from build123d import *

# Parameters (mm, degrees)
SKETCH1_W           = 304.8
SKETCH1_H           = 50.8
SKETCH1_R           = 2.6
SKETCH1_R_2         = 4.05
BOSS_EXTRUDE1_DEPTH = 3.175


with BuildPart() as part:
    # Sketch1 → Boss-Extrude1 (new body)
    with BuildSketch(Plane(origin=(0, 0, 0), x_dir=(1, 0, 0), z_dir=(0, 1, 0))):
        with Locations((152.4, 25.4)):
            Rectangle(SKETCH1_W, SKETCH1_H)
        with Locations(Location((19.185127899, 44.45, 0), (0, 0, 270))):
            Circle(SKETCH1_R, mode=Mode.SUBTRACT)
        with Locations(Location((19.185127899, 20, 0), (0, 0, 270))):
            Circle(SKETCH1_R_2, mode=Mode.SUBTRACT)
        with Locations(Location((99.185127899, 20, 0), (0, 0, 270))):
            Circle(SKETCH1_R_2, mode=Mode.SUBTRACT)
        with Locations(Location((99.185127899, 44.45, 0), (0, 0, 270))):
            Circle(SKETCH1_R, mode=Mode.SUBTRACT)
        with Locations(Location((179.185127899, 20, 0), (0, 0, 270))):
            Circle(SKETCH1_R_2, mode=Mode.SUBTRACT)
        with Locations(Location((179.185127899, 44.45, 0), (0, 0, 270))):
            Circle(SKETCH1_R, mode=Mode.SUBTRACT)
        with Locations(Location((259.185127899, 20, 0), (0, 0, 270))):
            Circle(SKETCH1_R_2, mode=Mode.SUBTRACT)
        with Locations(Location((259.185127899, 44.45, 0), (0, 0, 270))):
            Circle(SKETCH1_R, mode=Mode.SUBTRACT)
    extrude(amount=BOSS_EXTRUDE1_DEPTH)


solid = part.part
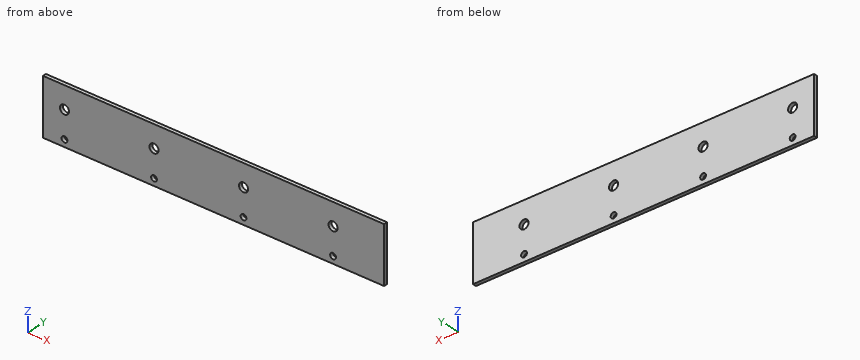
Read the model definition and answer for the solid it produces. Units are mm, in the model's axes. Coordinates: 2 decimals unless noted, no trailing zeros. Loops run counter-clockwise (first coordinate to the right, second up) from the corner with the lowest first, then second, coordinate; pieces in that order, holes last. Notation, with made-up numbers: (-8.5, 61) -> (-0.5, 61) arc R21 ccw to (-0.5, 82) -> close; hole circle Ø2 at (37.25, 9). An arc over 180 degrees is marked (long way). Answer in a Markdown table with one row per item.
Item 1: A cutting plane is placed at A-A on z = -44.45. Determine the outline of the cut face in (x, y) (3 decimals), plus the area to 3 significant figures.
Returned:
| item | result |
|---|---|
| outline | (0, 0) -> (16.585, 0) -> (16.585, 3.175) -> (0, 3.175) -> close; (21.785, 0) -> (96.585, 0) -> (96.585, 3.175) -> (21.785, 3.175) -> close; (101.785, 0) -> (176.585, 0) -> (176.585, 3.175) -> (101.785, 3.175) -> close; (181.785, 0) -> (256.585, 0) -> (256.585, 3.175) -> (181.785, 3.175) -> close; (261.785, 0) -> (304.8, 0) -> (304.8, 3.175) -> (261.785, 3.175) -> close |
| area | 902 mm^2 |
Item 2: A cutting plane is placed at C-C on z = -20. Determine the outline of the cut face in (x, y) (3 decimals).
Returned:
| item | result |
|---|---|
| outline | (0, 0) -> (15.135, 0) -> (15.135, 3.175) -> (0, 3.175) -> close; (23.235, 0) -> (95.135, 0) -> (95.135, 3.175) -> (23.235, 3.175) -> close; (103.235, 0) -> (175.135, 0) -> (175.135, 3.175) -> (103.235, 3.175) -> close; (183.235, 0) -> (255.135, 0) -> (255.135, 3.175) -> (183.235, 3.175) -> close; (263.235, 0) -> (304.8, 0) -> (304.8, 3.175) -> (263.235, 3.175) -> close |
Item 3: A cutting plane is placed at B-B on y = 1.8. Give the number of separate pieces and of enclosed holes in the cut face, plus the area to 3 significant figures.
Returned:
| item | result |
|---|---|
| separate pieces | 1 |
| enclosed holes | 8 |
| area | 15,200 mm^2 |
Item 4: Each of these flat-tipped pins is pushed along its axis until it touches: P1, Ø8.5, axis at x = 179.19, z = -44.45, coming from the -Y side; P2, Ø7.5, axis at x = 19.19, z = -20, coming from the +Y side. Where does it stop, or does it pass through?
Returned:
| item | result |
|---|---|
| P1 | stops at y = 0 |
| P2 | passes through |
Item 5: Straight lines are drawn through the part: line 1 along X through (y, z) = (1.7, -44.45); line 2 along X through (y, z) = (2.1, -20). For each, find the intervals that lie inside material, in ascending order. Write a range as [from, to].
Returned:
| item | result |
|---|---|
| line 1 | x = [0, 16.59], [21.79, 96.59], [101.79, 176.59], [181.79, 256.59], [261.79, 304.8] |
| line 2 | x = [0, 15.14], [23.24, 95.14], [103.24, 175.14], [183.24, 255.14], [263.24, 304.8] |
